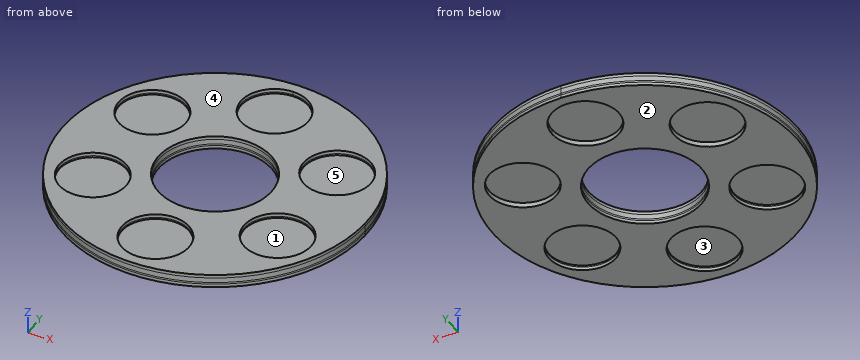
from build123d import *

# Parameters (mm, degrees)
F0_R         = 16.025
F0_R_2       = 27
F1_DEPTH     = 2.3815
F1_FACE_R    = 16.025
F1_FACE_R_2  = 27
F1_FACE1_R   = 16.025
F1_FACE1_R_2 = 27
F2_DEPTH     = 1.56


with BuildPart() as f1:
    # F0 (on Top) → F1 (new body, symmetric)
    with BuildSketch(Plane.XY):
        with BuildLine():
            ThreePointArc((0, 72.5), (-51.265241636, -51.265241636), (72.5, 0))
            ThreePointArc((72.5, 0), (51.265241636, 51.265241636), (0, 72.5))
        make_face()
        with Locations((-44.6003082949, -25.75)):
            Circle(F0_R, mode=Mode.SUBTRACT)
        with Locations((0, -51.5)):
            Circle(F0_R, mode=Mode.SUBTRACT)
        with Locations((44.6003082949, -25.75)):
            Circle(F0_R, mode=Mode.SUBTRACT)
        with Locations((-44.6003082949, 25.75)):
            Circle(F0_R, mode=Mode.SUBTRACT)
        Circle(F0_R_2, mode=Mode.SUBTRACT)
        with Locations((44.6003082949, 25.75)):
            Circle(F0_R, mode=Mode.SUBTRACT)
        with BuildLine():
            ThreePointArc((16.025, 51.5), (-11.3313861685, 40.1686138315), (0, 67.525))
            ThreePointArc((0, 67.525), (11.3313861685, 62.8313861685), (16.025, 51.5))
        make_face(mode=Mode.SUBTRACT)
    extrude(amount=F1_DEPTH, both=True)

    # F0 (on Top) + F1_face (on face) + F1_face1 (on face) → F2 (join)
    with BuildSketch(Plane.XY):
        with Locations((-44.6003082949, 25.75)):
            Circle(F0_R)
        with BuildLine():
            ThreePointArc((16.025, 51.5), (11.3313861685, 62.8313861685), (0, 67.525))
            ThreePointArc((0, 67.525), (-11.3313861685, 40.1686138315), (16.025, 51.5))
        make_face()
        with Locations((44.6003082949, 25.75)):
            Circle(F0_R)
        with Locations((44.6003082949, -25.75)):
            Circle(F0_R)
        with Locations((0, -51.5)):
            Circle(F0_R)
        with Locations((-44.6003082949, -25.75)):
            Circle(F0_R)
    with BuildSketch(Plane.XY.offset(2.3815)):
        with BuildLine():
            ThreePointArc((72.5, 0), (51.265241636, 51.265241636), (0, 72.5))
            ThreePointArc((0, 72.5), (-51.265241636, -51.265241636), (72.5, 0))
        make_face()
        with Locations((-44.6003082949, -25.75)):
            Circle(F1_FACE_R, mode=Mode.SUBTRACT)
        with Locations((0, -51.5)):
            Circle(F1_FACE_R, mode=Mode.SUBTRACT)
        with Locations((44.6003082949, -25.75)):
            Circle(F1_FACE_R, mode=Mode.SUBTRACT)
        with Locations((-44.6003082949, 25.75)):
            Circle(F1_FACE_R, mode=Mode.SUBTRACT)
        Circle(F1_FACE_R_2, mode=Mode.SUBTRACT)
        with Locations((44.6003082949, 25.75)):
            Circle(F1_FACE_R, mode=Mode.SUBTRACT)
        with BuildLine():
            ThreePointArc((16.025, 51.5), (-11.3313861685, 40.1686138315), (0, 67.525))
            ThreePointArc((0, 67.525), (11.3313861685, 62.8313861685), (16.025, 51.5))
        make_face(mode=Mode.SUBTRACT)
    with BuildSketch(Plane(origin=(0, 0, -2.3815), x_dir=(1, 0, 0), z_dir=(0, 0, -1))):
        with BuildLine():
            ThreePointArc((0, -72.5), (51.265241636, -51.265241636), (72.5, 0))
            ThreePointArc((72.5, 0), (-51.265241636, 51.265241636), (0, -72.5))
        make_face()
        with Locations((-44.6003082949, 25.75)):
            Circle(F1_FACE1_R, mode=Mode.SUBTRACT)
        with Locations((0, 51.5)):
            Circle(F1_FACE1_R, mode=Mode.SUBTRACT)
        with Locations((44.6003082949, 25.75)):
            Circle(F1_FACE1_R, mode=Mode.SUBTRACT)
        with Locations((-44.6003082949, -25.75)):
            Circle(F1_FACE1_R, mode=Mode.SUBTRACT)
        Circle(F1_FACE1_R_2, mode=Mode.SUBTRACT)
        with Locations((44.6003082949, -25.75)):
            Circle(F1_FACE1_R, mode=Mode.SUBTRACT)
        with BuildLine():
            ThreePointArc((0, -67.525), (-11.3313861685, -40.1686138315), (16.025, -51.5))
            ThreePointArc((16.025, -51.5), (11.3313861685, -62.8313861685), (0, -67.525))
        make_face(mode=Mode.SUBTRACT)
    extrude(amount=F2_DEPTH, dir=(0, 0, 1))


solid = f1.part
Verification items for the finished model (mm, model axes). Face numbers are marked on the shaded views. A direction names the side the tool comes from. Round coordinates to 2 decimals unless told otherwise and drop trailing zeros. Order: outer loops, then holes, each group sorted by start corner. A loop starts at its lowest first (then second) coordinate and runs counter-clockwise, first axis right, second up.
1. Thickness scan on L1, parallel to X at y = -22.5, z = -1; L2, parallel to X at y = -28.5, z = -1; L3, parallel to Y at x = 5, z = -0.25 (3 decimals). Record the ranges inside material, lowest first.
Final values:
L1: x = -68.92 to -60.29, -28.91 to -14.92, 14.92 to 28.91, 60.29 to 68.92
L2: x = -66.66 to -60.39, -28.81 to 28.81, 60.39 to 66.66
L3: y = -72.327 to -66.725, -36.275 to -26.533, 26.533 to 36.275, 66.725 to 72.327
2. Access from +Z, -Z, +X, -X, +Y, -Y to the whole of each face (thin tool, end or side, straight path). Record for the marked faces 3, 4 and 5.
Final values:
face 3: -Z
face 4: +Z, +X, -X, +Y, -Y
face 5: +Z
3. Section check B-B on y = -19. Record the cut outline in (x, z), then the cut area to 3 significant figures.
Final values:
outline: (-69.97, -2.38) - (-59.13, -2.38) - (-59.13, 0) - (-30.07, 0) - (-30.07, -2.38) - (-19.18, -2.38) - (-19.18, 3.94) - (-30.07, 3.94) - (-30.07, 1.56) - (-59.13, 1.56) - (-59.13, 3.94) - (-69.97, 3.94) - close; (19.18, -2.38) - (30.07, -2.38) - (30.07, 0) - (59.13, 0) - (59.13, -2.38) - (69.97, -2.38) - (69.97, 3.94) - (59.13, 3.94) - (59.13, 1.56) - (30.07, 1.56) - (30.07, 3.94) - (19.18, 3.94) - close
area: 365 mm2
4. Release check for a two-part mould opening along X. For the marked faces 1 and 2 record: +X half, -X half, draft (parallel to the pull), parting line (faces both ways), or undercut.
Final values:
face 1: undercut
face 2: draft
5. Go/stop test with flat-tipped pins: P1, Ø2, axis at y = 23.5, z = 1, coming from the -X side; P2, Ø19, axis at x = 44.6, y = -25.75, coming from the +Z side; P3, Ø19, axis at x = 0, y = 51.5, coming from the -Z side. Record where each tip stops, or that it passes through.
Final values:
P1: stops at x = -68.92
P2: stops at z = 1.56
P3: stops at z = 0
6. Section check A-A on x = 11.5. Record the cut outline in (y, z).
Final values:
outline: (-71.58, -2.38) - (-62.66, -2.38) - (-62.66, 0) - (-40.34, 0) - (-40.34, -2.38) - (-24.43, -2.38) - (-24.43, 3.94) - (-40.34, 3.94) - (-40.34, 1.56) - (-62.66, 1.56) - (-62.66, 3.94) - (-71.58, 3.94) - close; (24.43, -2.38) - (40.34, -2.38) - (40.34, 0) - (62.66, 0) - (62.66, -2.38) - (71.58, -2.38) - (71.58, 3.94) - (62.66, 3.94) - (62.66, 1.56) - (40.34, 1.56) - (40.34, 3.94) - (24.43, 3.94) - close
7. Section check C-C on x = 52.5. Record the cut outline in (y, z).
Final values:
outline: (-50, -2.38) - (-39.69, -2.38) - (-39.69, 0) - (-11.81, 0) - (-11.81, -2.38) - (11.81, -2.38) - (11.81, 0) - (39.69, 0) - (39.69, -2.38) - (50, -2.38) - (50, 3.94) - (39.69, 3.94) - (39.69, 1.56) - (11.81, 1.56) - (11.81, 3.94) - (-11.81, 3.94) - (-11.81, 1.56) - (-39.69, 1.56) - (-39.69, 3.94) - (-50, 3.94) - close
8. Section check D-D on y = 39. Record the cut outline in (x, z).
Final values:
outline: (-61.12, -2.38) - (-53.61, -2.38) - (-53.61, 0) - (-35.59, 0) - (-35.59, -2.38) - (-10.03, -2.38) - (-10.03, 0) - (10.03, 0) - (10.03, -2.38) - (35.59, -2.38) - (35.59, 0) - (53.61, 0) - (53.61, -2.38) - (61.12, -2.38) - (61.12, 3.94) - (53.61, 3.94) - (53.61, 1.56) - (35.59, 1.56) - (35.59, 3.94) - (10.03, 3.94) - (10.03, 1.56) - (-10.03, 1.56) - (-10.03, 3.94) - (-35.59, 3.94) - (-35.59, 1.56) - (-53.61, 1.56) - (-53.61, 3.94) - (-61.12, 3.94) - close
